Here's how the part is built. I have some questions about the finished solid (model axes, mm). A direction names the side the tool comes from. Coordinates: 2 decimals unless noted, no trailing zeros. Loops run counter-clockwise (first coordinate to the right, second up) from the corner with the lowest first, then second, coordinate; pieces in that order, holes last. Notation, with made-up numbers: (78, 32.25) -> (109, 32.25) arc R22 cw to (109, 64.25) -> close; hole circle Ø11 at (-31, -29). An arc over 180 degrees is marked (long way). Answer as a JSON object with one key per item and string values. Group by question number.
Q1. I want a section at C-C on y = 9.75. Write out the boundary of the cut face in (x, z), then the cut area to 3 significant figures.
Q2. On a 3-axis mill with a long thin cutter (end or side, diameter ignored), from which of +Z, -Z, +X, -X, +Y, -Y can I reach the whole of each face in a straight line? I mean faces 1 (the cylindrical face through (-6.1, 6.05, -2.53)), 2 (the cylindrical face through (1.22, 1.2, 9.32)). Say none if no direction works.
Q3. Thinking about a two-plate mould opening in Y: for faces 3 (the flat face through (0, 12.7, 0)), 4 (the cylindrical face through (1.22, 9.5, 9.32)), 5 (the flat face through (0, 0, 0)), 6 (the conical face through (5.348, 4.306, -4.101)), which applies, released by +Y, released by -Y, zero draft, split by the parting line, or undercut?
Q4. I need wall thicknesses on line 1 (Y direction, x = -6, z = 4.5); line 2 (Y direction, x = 1.25, z = -8.25); line 3 (Z direction, x = 0, y = 6.25). Which ranges of each line are inside material? Lowest first, please.
Q5. I want a section at A-A on z = 0. Write out the boundary of the cut face in (x, y) (1 decimal), then the cut area to 3 significant figures.
Q6. I'm going to push flat-ended pins straight in: pin 1 (4 mm diameter, centred on x = -2.5, y = 8, fed in from +Z); pin 2 (2 mm diameter, centred on y = 10, z = 4.5, fed in from -X); pin 3 (1.5 mm diameter, centred on y = 10.5, z = 5, fed in from +X). Where does each tip first touch, or does it pass through?
Q7. I want a section at D-D on y = 12.25. Write out the boundary of the cut face in (x, z).
Q8. I want a section at B-B on x = 0. Write out the boundary of the cut face in (y, z) (1 decimal), then the cut area to 3 significant figures.
```python
from build123d import *

# Parameters (mm, degrees)
FILLET1_R      = 0.79375
CHAMFER1_SIZE  = 0.79375
CHAMFER1_SIZE2 = 1.374815329


with BuildPart() as part:
    # Sketch1 → Revolve1 (revolve)
    with BuildSketch(Plane.XY):
        Polygon((0, 0), (-9.398, 0), (-9.398, 1.5875), (-6.604, 4.445), (-6.604, 7.62), (-9.398, 7.62), (-9.398, 12.7), (0, 12.7), align=None)
    revolve(axis=Axis((0, 0, 0), (0, 1, 0)))

    # Fillet1
    fillet1_edges = [part.edges().sort_by_distance(p)[0] for p in [
        (9.398, 0, 0),
    ]]
    fillet(fillet1_edges, radius=FILLET1_R)

    # Chamfer1
    chamfer1_edges = [part.edges().sort_by_distance(p)[0] for p in [
        (9.398, 12.7, 0),
    ]]
    chamfer1_side = [part.faces().sort_by_distance(p)[0] for p in [
        (0, 12.7, 0),
    ]]
    chamfer(chamfer1_edges, length=CHAMFER1_SIZE, length2=CHAMFER1_SIZE2, reference=chamfer1_side[0])


solid = part.part
```
Result set:
{
 "1": {"outline": "circle Ø18.8 at (0, 0)", "area": "277 mm²"},
 "2": {"face 1": "none", "face 2": "+Y, -Y"},
 "3": {"face 3": "released by +Y", "face 4": "zero draft", "face 5": "released by -Y", "face 6": "undercut"},
 "4": {"line 1": "y = 0 to 3.53, 7.62 to 12.7", "line 2": "y = 0 to 2.67, 7.62 to 12.7", "line 3": "z = -6.6 to 6.6"},
 "5": {"outline": "(-9.4, 0.8) arc R0.8 ccw to (-8.6, 0) -> (8.6, 0) arc R0.8 ccw to (9.4, 0.8) -> (9.4, 1.6) -> (6.6, 4.4) -> (6.6, 7.6) -> (9.4, 7.6) -> (9.4, 11.3) -> (8.6, 12.7) -> (-8.6, 12.7) -> (-9.4, 11.3) -> (-9.4, 7.6) -> (-6.6, 7.6) -> (-6.6, 4.4) -> (-9.4, 1.6) -> close", "area": "212 mm²"},
 "6": {"pin 1": "stops at z = 9.38", "pin 2": "stops at x = -8.72", "pin 3": "stops at x = 8.38"},
 "7": {"outline": "circle Ø17.73 at (0, 0)"},
 "8": {"outline": "(0, -8.6) arc R0.8 ccw to (0.8, -9.4) -> (1.6, -9.4) -> (4.4, -6.6) -> (7.6, -6.6) -> (7.6, -9.4) -> (11.3, -9.4) -> (12.7, -8.6) -> (12.7, 8.6) -> (11.3, 9.4) -> (7.6, 9.4) -> (7.6, 6.6) -> (4.4, 6.6) -> (1.6, 9.4) -> (0.8, 9.4) arc R0.8 ccw to (0, 8.6) -> close", "area": "212 mm²"}
}
